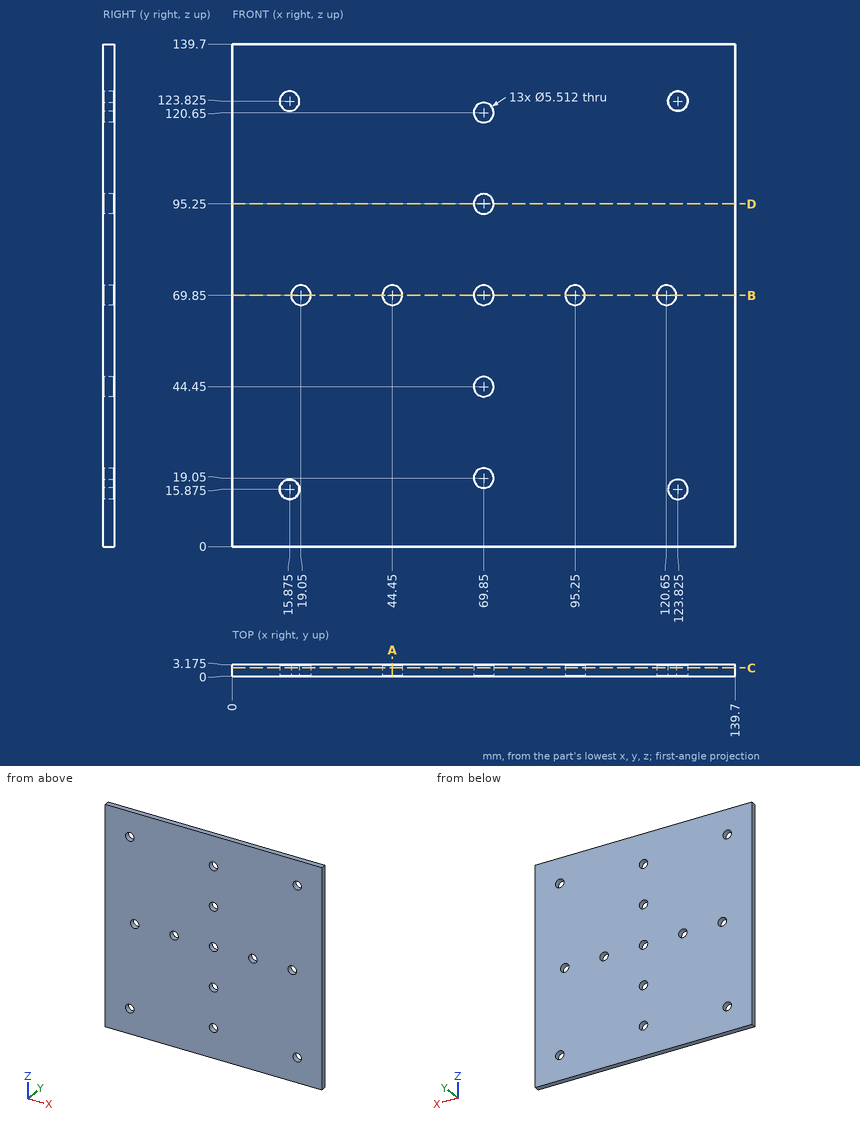
Source: three-view drawing plus pictorial views. Frame: mm from the lowest corner of the part. Coordinates: 2 decimals unless noted, no trailing zeros. Loops run counter-clockwise (first coordinate to the right, second up) from the corner with the lowest first, then second, coordinate; pieces in that order, holes last. Notation, with made-up numbers: (11.25, 33) - (36.25, 33) arc R31 cw to (36.25, 62) - close; hole circle Ø8 at (-11.75, 67.25). An arc over 180 degrees is marked (long way). Answer in a Markdown table with one row per item. Add a question column.
Item 1: Contact query for a flat-ended pin moving along its axis: P1, Ø7, axis at x = 69.85, z = 120.65, coming from the -Y side. Output: stop coordinate, or through.
Item 2: Section query B-B on z = 69.85. Return the cut outline in (x, y) (1 decimal).
Item 3: Section query A-A on x = 44.45. Return the cut outline in (y, z) (1 decimal).
Item 4: Line query: line 1 along Z through (x, y) = (69.85, 2.35); line 2 along X through (y, z) = (0.75, 19.05). Output: solid intervals per line, ascending. Write a range as [from, to].
Item 5: Section query D-D on z = 95.25. Return the cut outline in (x, y) (1 decimal), then the cut area to 3 significant figures.
Item 6: Section query C-C on y = 2.25. State how many separate pieces and enclosed holes the cut face has, then the cut area to 3 significant figures.
Recorded:
| question | item | result |
|---|---|---|
| 1 | P1 | y = 0 |
| 2 | outline | (0, 0) - (16.3, 0) - (16.3, 3.2) - (0, 3.2) - close; (21.8, 0) - (41.7, 0) - (41.7, 3.2) - (21.8, 3.2) - close; (47.2, 0) - (67.1, 0) - (67.1, 3.2) - (47.2, 3.2) - close; (72.6, 0) - (92.5, 0) - (92.5, 3.2) - (72.6, 3.2) - close; (98, 0) - (117.9, 0) - (117.9, 3.2) - (98, 3.2) - close; (123.4, 0) - (139.7, 0) - (139.7, 3.2) - (123.4, 3.2) - close |
| 3 | outline | (0, 0) - (3.2, 0) - (3.2, 67.1) - (0, 67.1) - close; (0, 72.6) - (3.2, 72.6) - (3.2, 139.7) - (0, 139.7) - close |
| 4 | line 1 | [0, 16.29], [21.81, 41.69], [47.21, 67.09], [72.61, 92.49], [98.01, 117.89], [123.41, 139.7] |
| 4 | line 2 | [0, 67.09], [72.61, 139.7] |
| 5 | outline | (0, 0) - (67.1, 0) - (67.1, 3.2) - (0, 3.2) - close; (72.6, 0) - (139.7, 0) - (139.7, 3.2) - (72.6, 3.2) - close |
| 5 | area | 426 mm^2 |
| 6 | separate pieces | 1 |
| 6 | enclosed holes | 13 |
| 6 | area | 19,200 mm^2 |
